The listing builds one solid part. Answer for the finished solid, in the listing's coordinates (mm). A direction names the side the tool comes from. Give positions to 0.01 mm unless a question says otherwise; leave off trailing zeros. Order: outer loops, then holes, each group sorted by start corner. A loop starts at its lowest first (then second) coordinate and runs counter-clockwise, first axis right, second up. Notation, with made-up numbers: (55.5, -13) -> (90.5, -13) arc R30 cw to (90.5, 16) -> close; hole circle Ø3 at (15, 88.5). An arc over 180 degrees is marked (long way). Write item = value, one per line. Start each with the question number.
```python
from build123d import *

# Parameters (mm, degrees)
SKETCH1_R           = 2.15
BOSS_EXTRUDE1_DEPTH = 2
SKETCH5_R           = 2.774437445
SKETCH5_R_2         = 13.25
BOSS_EXTRUDE2_DEPTH = 2


with BuildPart() as part:
    # Sketch1 → Boss-Extrude1 (new body)
    with BuildSketch(Plane(origin=(0, 0, 0), x_dir=(1, 0, 0), z_dir=(0, 1, 0))):
        with BuildLine():
            Line((-26.604565316, -31.465), (26.604565316, -31.465))
            ThreePointArc((26.604565316, -31.465), (29.005500206, -30.470500206), (30, -28.069565316))
            Line((30, -28.069565316), (30, 31.465))
            Line((30, 31.465), (-30, 31.465))
            Line((-30, 31.465), (-30, -28.069565316))
            ThreePointArc((-30, -28.069565316), (-29.005500206, -30.470500206), (-26.604565316, -31.465))
        make_face()
        with Locations(Location((-23, -25.135, 0), (0, 0, 270))):
            Circle(SKETCH1_R, mode=Mode.SUBTRACT)
        with Locations(Location((-23, 17.465, 0), (0, 0, 270))):
            Circle(SKETCH1_R, mode=Mode.SUBTRACT)
        with Locations(Location((23, -25.135, 0), (0, 0, 90))):
            Circle(SKETCH1_R, mode=Mode.SUBTRACT)
        with Locations(Location((23, 17.465, 0), (0, 0, 90))):
            Circle(SKETCH1_R, mode=Mode.SUBTRACT)
        with BuildLine():
            Line((-12.5, 19.838201533), (12.5, 19.838201533))
            ThreePointArc((12.5, 19.838201533), (14.65, 17.688201533), (12.5, 15.538201533))
            Line((12.5, 15.538201533), (-12.5, 15.538201533))
            ThreePointArc((-12.5, 15.538201533), (-14.65, 17.688201533), (-12.5, 19.838201533))
        make_face(mode=Mode.SUBTRACT)
        with BuildLine():
            Line((-20.85, 9.615), (-20.85, 5.315))
            ThreePointArc((-20.85, 5.315), (-23, 3.165), (-25.15, 5.315))
            Line((-25.15, 5.315), (-25.15, 9.615))
            ThreePointArc((-25.15, 9.615), (-23, 11.765), (-20.85, 9.615))
        make_face(mode=Mode.SUBTRACT)
        with BuildLine():
            Line((-20.85, -9.685), (-20.85, -13.985))
            ThreePointArc((-20.85, -13.985), (-23, -16.135), (-25.15, -13.985))
            Line((-25.15, -13.985), (-25.15, -9.685))
            ThreePointArc((-25.15, -9.685), (-23, -7.535), (-20.85, -9.685))
        make_face(mode=Mode.SUBTRACT)
        with BuildLine():
            Line((-12.5, -10.835), (12.5, -10.835))
            ThreePointArc((12.5, -10.835), (14.65, -12.985), (12.5, -15.135))
            Line((12.5, -15.135), (-12.5, -15.135))
            ThreePointArc((-12.5, -15.135), (-14.65, -12.985), (-12.5, -10.835))
        make_face(mode=Mode.SUBTRACT)
        with BuildLine():
            Line((20.85, -9.685), (20.85, -13.985))
            ThreePointArc((20.85, -13.985), (23, -16.135), (25.15, -13.985))
            Line((25.15, -13.985), (25.15, -9.685))
            ThreePointArc((25.15, -9.685), (23, -7.535), (20.85, -9.685))
        make_face(mode=Mode.SUBTRACT)
        with BuildLine():
            Line((20.85, 9.615), (20.85, 5.315))
            ThreePointArc((20.85, 5.315), (23, 3.165), (25.15, 5.315))
            Line((25.15, 5.315), (25.15, 9.615))
            ThreePointArc((25.15, 9.615), (23, 11.765), (20.85, 9.615))
        make_face(mode=Mode.SUBTRACT)
    extrude(amount=BOSS_EXTRUDE1_DEPTH)

    # Sketch5 → Boss-Extrude2 (add)
    with BuildSketch(Plane(origin=(0, 0, -31.465), x_dir=(-1, 0, 0), z_dir=(0, 0, -1))):
        with BuildLine():
            ThreePointArc((-30, 32), (0, 62), (30, 32))
            Line((30, 32), (30, 2))
            Line((30, 2), (-30, 2))
            Line((-30, 2), (-30, 32))
        make_face()
        with Locations((12.374368671, 19.625631329)):
            Circle(SKETCH5_R, mode=Mode.SUBTRACT)
        with Locations((-12.374368671, 19.625631329)):
            Circle(SKETCH5_R, mode=Mode.SUBTRACT)
        with Locations((-12.374368671, 44.374368671)):
            Circle(SKETCH5_R, mode=Mode.SUBTRACT)
        with Locations((12.374368671, 44.374368671)):
            Circle(SKETCH5_R, mode=Mode.SUBTRACT)
        with Locations((0, 32)):
            Circle(SKETCH5_R_2, mode=Mode.SUBTRACT)
    extrude(amount=-BOSS_EXTRUDE2_DEPTH)


solid = part.part
```
Item 1: Which of the six approach directions +Z, -Z, +X, -X, +Y, -Y give full straight-line access (tool end or side, diameter ignored) to faces 1 (the flat face through (6, 19, -29.465)), 2 (the flat face through (0, 1, -19.838)), 3 (the cylindrical face through (-29.032, 0.986, 30.444))?
Item 2: Consider L1, parallel to Z at x = 23, y = 1.3 (3 decimals); L2, parallel to Y at x = 0, z = -30.7; L3, parallel to Z at x = -6, y = 13.5 (3 decimals). Determine where each line is inside the solid, lowest interval first. Write a range as from..to.
Item 3: A cutting plane is placed at A-A, the plane x = 0. Write down the section's boundary in (y, z) (3 decimals), plus the area to 3 significant figures.
Item 4: Flat-ended cylindrical pins translate along their axes: pin 1 (6 mm diameter, centred on x = 7.5, z = -23, fed in from +Y); pin 2 (3.5 mm diameter, centred on x = 12.37, y = 44.37, fed in from +Z); pin 3 (1.5 mm diameter, centred on x = 8.5, y = 7, fed in from +Z) (3 decimals). Find the tip coordinate at first contact, or state that the pin passes through.
Item 5: A cutting plane is placed at D-D, the plane z = 6.5. Write down the section's boundary in (x, y).
Item 6: A cutting plane is placed at C-C, the plane x = -23. Write down the section's boundary in (y, z) (3 decimals).
Item 7: The mould has two halves that part along Y. Classify faces 4 (the flat face through (30, 1.7, -10.7)), 5 (the flat face through (0, 2, 1)), 6 (the cylindrical face through (-6.114, 20.245, -30.479)): +Y half, -Y half, draft (parallel to the pull), parting line (faces both ways), or undercut.
Item 8: A cutting plane is placed at B-B, the plane y = 29. Write down the section's boundary in (x, z) (3 decimals), plus the area to 3 significant figures.
Check values:
q1.face_1 = +Z, +X, -X, +Y
q1.face_2 = +Y, -Y
q1.face_3 = +Z, -X, +Y, -Y
q2.L1 = -31.465..-19.615, -15.315..-11.765, -3.165..7.535, 16.135..22.985, 27.285..31.465
q2.L2 = 0..18.75, 45.25..62
q2.L3 = -31.465..-29.465
q3.outline = (0, -31.465) -> (18.75, -31.465) -> (18.75, -29.465) -> (2, -29.465) -> (2, -19.838) -> (0, -19.838) -> close; (0, -15.538) -> (2, -15.538) -> (2, 10.835) -> (0, 10.835) -> close; (0, 15.135) -> (2, 15.135) -> (2, 31.465) -> (0, 31.465) -> close; (45.25, -31.465) -> (62, -31.465) -> (62, -29.465) -> (45.25, -29.465) -> close
q3.area = 176 mm^2
q4.pin_1 = 2
q4.pin_2 = through
q4.pin_3 = -29.465
q5.outline = (-30, 0) -> (30, 0) -> (30, 2) -> (-30, 2) -> close
q6.outline = (0, -31.465) -> (51.261, -31.465) -> (51.261, -29.465) -> (2, -29.465) -> (2, -19.615) -> (0, -19.615) -> close; (0, -15.315) -> (2, -15.315) -> (2, -11.765) -> (0, -11.765) -> close; (0, -3.165) -> (2, -3.165) -> (2, 7.535) -> (0, 7.535) -> close; (0, 16.135) -> (2, 16.135) -> (2, 22.985) -> (0, 22.985) -> close; (0, 27.285) -> (2, 27.285) -> (2, 31.465) -> (0, 31.465) -> close
q7.face_4 = draft
q7.face_5 = +Y half
q7.face_6 = undercut
q8.outline = (-30, -31.465) -> (-12.906, -31.465) -> (-12.906, -29.465) -> (-30, -29.465) -> close; (12.906, -31.465) -> (30, -31.465) -> (30, -29.465) -> (12.906, -29.465) -> close
q8.area = 68.4 mm^2
